from build123d import *

# Parameters (mm, degrees)
SKETCH_2_R      = 2.5
EXTRUDE_2_DEPTH = 5
SKETCH_3_R      = 4
EXTRUDE_4_DEPTH = 5


with BuildPart() as part:
    # Эскиз2 → Бобышка-Вытянуть2 (new body)
    with BuildSketch(Plane.XY.offset(31.602998)):
        with BuildLine():
            Line((0, 3.5), (-0.979795897, 2.3))
            ThreePointArc((-0.979795897, 2.3), (0, 2.5), (0.979795897, 2.3))
            Line((0.979795897, 2.3), (0, 3.5))
        make_face()
        with BuildLine():
            Line((3.031088913, 1.75), (1.50196048, 1.998528137))
            ThreePointArc((1.50196048, 1.998528137), (2.165063509, 1.25), (2.481756377, 0.301471863))
            Line((2.481756377, 0.301471863), (3.031088913, 1.75))
        make_face()
        with BuildLine():
            Line((3.031088913, -1.75), (2.481756377, -0.301471863))
            ThreePointArc((2.481756377, -0.301471863), (2.165063509, -1.25), (1.50196048, -1.998528137))
            Line((1.50196048, -1.998528137), (3.031088913, -1.75))
        make_face()
        with BuildLine():
            ThreePointArc((0.979795897, -2.3), (0, -2.5), (-0.979795897, -2.3))
            Line((-0.979795897, -2.3), (0, -3.5))
            Line((0, -3.5), (0.979795897, -2.3))
        make_face()
        with BuildLine():
            ThreePointArc((-2.481756377, 0.301471863), (-2.165063509, 1.25), (-1.50196048, 1.998528137))
            Line((-1.50196048, 1.998528137), (-3.031088913, 1.75))
            Line((-3.031088913, 1.75), (-2.481756377, 0.301471863))
        make_face()
        with BuildLine():
            ThreePointArc((-1.50196048, -1.998528137), (-2.165063509, -1.25), (-2.481756377, -0.301471863))
            Line((-2.481756377, -0.301471863), (-3.031088913, -1.75))
            Line((-3.031088913, -1.75), (-1.50196048, -1.998528137))
        make_face()
        Circle(SKETCH_2_R)
    extrude(amount=EXTRUDE_2_DEPTH)

    # Эскиз3 → Бобышка-Вытянуть4 (add)
    with BuildSketch(Plane.XY.offset(31.602998)):
        Circle(SKETCH_3_R)
    extrude(amount=-EXTRUDE_4_DEPTH)


solid = part.part
Design review of the part built by this model. Coordinates are the model's own, in mm. A direction names the side the tool comes from. Round coordinates to 2 decimals unless told otherwise and drop trailing zeros. Write each loop counter-clockwise with the first axis right and the second up, starting at its lowest first coordinate (ties: lowest second). Pieces come first, ordered by that corner, then holes. Notation, with made-up numbers: (-6, -40) -> (35, -40) arc R25 ccw to (35, -19) -> close; hole circle Ø4 at (1, 89). An arc over 180 degrees is marked (long way). One line per item, written item: value. Start each with the question number.
Q1. Add section D-D (x = 2.75). Give the boundary of the cut face in (y, z).
Q2. Insertion check: P1, Ø1.5, axis at x = 3, z = 35, coming from the +Y side; P2, Ø2, axis at x = 2, z = 28.5, coming from the +Y side; P3, Ø3, axis at x = 0, z = 35, coming from the +Y side. Each pin has a flat end and moves straight along its axis. Give the tip position at first contact, or say it passes through.
Q3. Tool access review of faces 1 (the face through (3, 0, 31.603)), 2 (the face through (2.753, 1.016, 34.068)), 3 (the face through (-2.753, -1.016, 34.068)), 4 (the face through (-0.5, -2.89, 34.07)), 5 (the face through (0.48, -2.91, 34.07)): name each direction out of +Z, -Z, +X, -X, +Y, -Y from which nothing blocks a thin tool from reaching the whole face with its end or side.
Q4. To check wall thickness, follow probe 1 along Z at (x, y) = (-2.5, -2.75); probe 2 along Y at (x, z) = (1, 27.75); probe 3 along X at (y, z) = (-3.25, 31.75). State the ranges of each line that lie inside material, in increasing order.
Q5. Add section C-C (x = -2). Give the boundary of the cut face in (y, z).
Q6. Add section A-A (z = 32.5). Give the boundary of the cut face in (x, y).
Q7. Add section B-B (y = 0). Give the boundary of the cut face in (x, z), then the cut area to 3 significant figures.
Q8. The part is to be moulded in two halves that separate along Y. For faces 6 (the face through (2.76, -1.04, 34.07)), 7 (the face through (-2.256, 1.876, 34.068)), 8 (the face through (-2.76, 1.04, 34.07)), 9 (the face through (-2.277, -1.873, 34.068)), say which applies: pulls with the +Y half, pulls with the -Y half, needs draft (parallel to the pull), parting line crosses it, or undercut.
Response:
1. outline: (-2.9, 26.6) -> (2.9, 26.6) -> (2.9, 31.6) -> (1.8, 31.6) -> (1.8, 36.6) -> (1.01, 36.6) -> (1.01, 31.6) -> (-1.01, 31.6) -> (-1.01, 36.6) -> (-1.8, 36.6) -> (-1.8, 31.6) -> (-2.9, 31.6) -> close
2. P1: stops at y = 1.88
2. P2: stops at y = 3.87
2. P3: stops at y = 3.5
3. face 1: +Z
3. face 2: +Z, +X
3. face 3: +Z, -X
3. face 4: +Z, -X, -Y
3. face 5: +Z, +X, -Y
4. probe 1: z = 26.6 to 31.6
4. probe 2: y = -3.87 to 3.87
4. probe 3: x = -0.2 to 0.2
5. outline: (-3.46, 26.6) -> (3.46, 26.6) -> (3.46, 31.6) -> (1.92, 31.6) -> (1.92, 36.6) -> (-1.92, 36.6) -> (-1.92, 31.6) -> (-3.46, 31.6) -> close
6. outline: (-3.03, -1.75) -> (-1.5, -2) arc R2.5 ccw to (-0.98, -2.3) -> (0, -3.5) -> (0.98, -2.3) arc R2.5 ccw to (1.5, -2) -> (3.03, -1.75) -> (2.48, -0.3) arc R2.5 ccw to (2.48, 0.3) -> (3.03, 1.75) -> (1.5, 2) arc R2.5 ccw to (0.98, 2.3) -> (0, 3.5) -> (-0.98, 2.3) arc R2.5 ccw to (-1.5, 2) -> (-3.03, 1.75) -> (-2.48, 0.3) arc R2.5 ccw to (-2.48, -0.3) -> close
7. outline: (-4, 26.6) -> (4, 26.6) -> (4, 31.6) -> (2.5, 31.6) -> (2.5, 36.6) -> (-2.5, 36.6) -> (-2.5, 31.6) -> (-4, 31.6) -> close
7. area: 65.0 mm^2
8. face 6: undercut
8. face 7: pulls with the +Y half
8. face 8: undercut
8. face 9: pulls with the -Y half
